Input: dimensioned drawing with shaded views. Units: mm. Origin: part minimum x, y, z. Round coordinates to 2 decimals unless told otherwise and drop trailing zeros. Order: outer loops, then holes, each group sorted by start corner. A loop starts at its lowest first (then second) coordinate and runs counter-clockwise, first axis right, second up. Notation, with made-up numbers: M 36,-15.75 L 81,-15.75 A14 ccw 81,-8.75 Z; hole C -21.5,24 d1. An arc over 180 degrees is marked long. Answer as CSV lines item,"result". Start each with the question number.
Item 1: Line query: line 1 (Z direction, x = 7, y = 1.7); line 2 (X direction, y = 1.8, z = 4) (1 decimal); line 3 (X direction, y = 1.55, z = 29) (1 decimal). Output: solid intervals per line, ascending. Write a range as [from, to].
Item 2: Section query B-B on y = 1.2. Return the cut outline in (x, z) (1 decimal), plus the area to 3 significant figures.
Item 3: Section query A-A on x = 7. Return the cut outline in (y, z).
Item 4: Pull-direction query (Z, two-part tool) for the marked faces 1, 2 and 3; classes: +Z half, -Z half, draft (parallel to the pull), parting line (faces both ways), or undercut.
Item 5: Section query C-C on z = 29. Return the cut outline in (x, y) (1 decimal).
Item 6: Section query D-D on z = 4. Return the cut outline in (x, y).
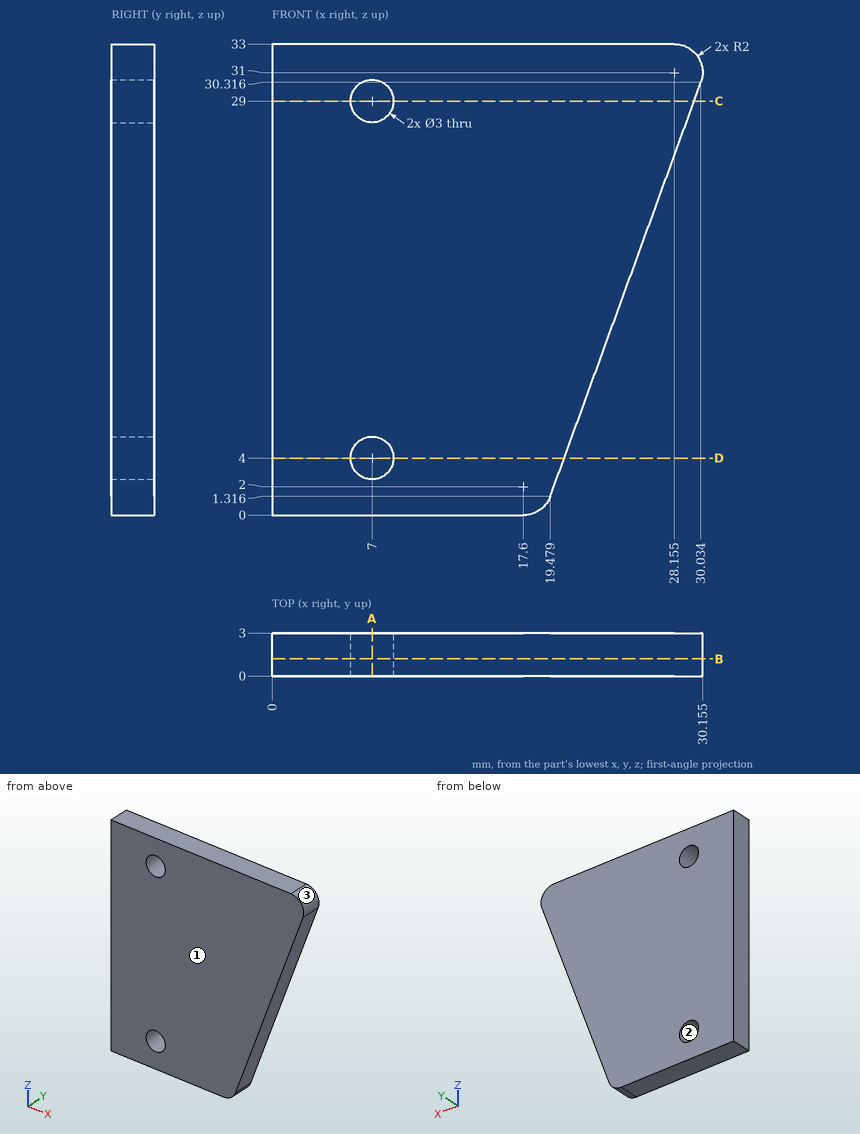
Results:
1,line 1,"[0, 2.5], [5.5, 27.5], [30.5, 33]"
1,line 2,"[0, 5.5], [8.5, 20.5]"
1,line 3,"[0, 5.5], [8.5, 29.6]"
2,outline,"M 0,0 L 17.6,0 A2 ccw 19.5,1.3 L 30,30.3 A2 ccw 28.2,33 L 0,33 Z; hole C 7,4 d3; hole C 7,29 d3"
2,area,"809 mm^2"
3,outline,"M 0,0 L 3,0 L 3,2.5 L 0,2.5 Z; M 0,5.5 L 3,5.5 L 3,27.5 L 0,27.5 Z; M 0,30.5 L 3,30.5 L 3,33 L 0,33 Z"
4,face 1,"draft"
4,face 2,"undercut"
4,face 3,"parting line"
5,outline,"M 0,0 L 5.5,0 L 5.5,3 L 0,3 Z; M 8.5,0 L 29.6,0 L 29.6,3 L 8.5,3 Z"
6,outline,"M 0,0 L 5.5,0 L 5.5,3 L 0,3 Z; M 8.5,0 L 20.46,0 L 20.46,3 L 8.5,3 Z"
